Input: part model. Units: mm. Frame: model coordinates. Face numbers are marked on the shaded views. A direction names the side the tool comes from. Give positions to 0.01 mm unless a question says otherwise; leave off trailing zeros. Loops run counter-clockwise (first coordinate to the right, second up) from the corner with the lowest first, then second, coordinate; pieces in that order, holes last. Notation, with made-up numbers: M -6.5,-16.5 L 40.5,-16.5 A25 cw 40.5,22.5 Z; hole C 69,-7 d3. An arc over 180 degrees is marked long. Answer as a JSON object with one key per item and string values. Group by question number.
1) First-contact query: P1, Ø1, axis at x = 7.5, y = 3.5, coming from the -Z side; P2, Ø2.5, axis at x = -12.5, z = 0, coming from the -Y side. Flat tips, straight axial feed; report the tip coordinate or a pass-through.
2) Section query A-A on x = -12.5. Return loops of the section in (y, z).
3) Ray query, L1, parallel to X at y = 2, z = 0; L2, parallel to X at y = 2.65, z = 1; L3, parallel to X at y = 1.55, z = -3. Return the intervals inside material, ascending.
4) Draft query along X for the marked faces 4 and 5. Return one class per face: +X half, -X half, draft (parallel to the pull), parting line (faces both ways), or undercut.
5) Access query for the marked faces 1, 2 and 3. Directions: +Z, -Z, +X, -X, +Y, -Y. A direction counts if a zero-diameter tool reaches every point of the face in a straight line with its end or side. Return the directions, or none.
6) Section query C-C on y = 2. Return loops of the section in (x, z), plus the area to 3 significant figures.
7) Section query D-D on z = 4.75. Return loops of the section in (x, y), plus the area to 3 significant figures.
8) Section query B-B on z = 0. Return loops of the section in (x, y).
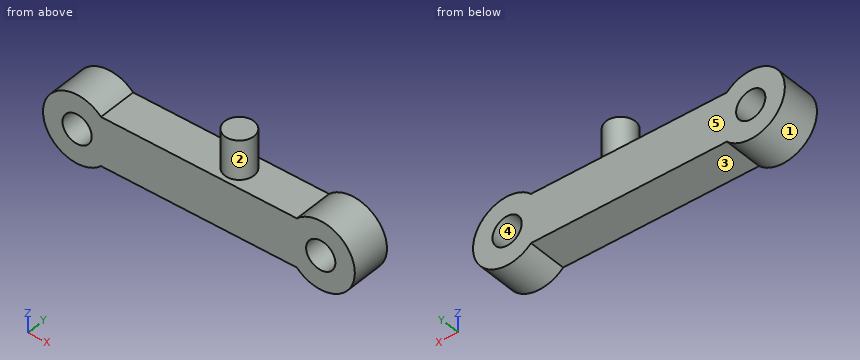
from build123d import *

# Parameters (mm, degrees)
SKETCH_1_R      = 1.5
EXTRUDE_1_DEPTH = 4
SKETCH_2_R      = 1.5
EXTRUDE_2_DEPTH = 4


with BuildPart() as part:
    # Эскиз1 → Бобышка-Вытянуть1 (new body)
    with BuildSketch(Plane(origin=(0, 0, 0), x_dir=(1, 0, 0), z_dir=(0, 1, 0))):
        with BuildLine():
            Line((-10.050510257, -2.5), (10.050510257, -2.5))
            ThreePointArc((10.050510257, -2.5), (16, 0), (10.050510257, 2.5))
            Line((10.050510257, 2.5), (-10.050510257, 2.5))
            ThreePointArc((-10.050510257, 2.5), (-16, 0), (-10.050510257, -2.5))
        make_face()
        with Locations(Location((-12.5, 0, 0), (0, 0, 270))):
            Circle(SKETCH_1_R, mode=Mode.SUBTRACT)
        with Locations(Location((12.5, 0, 0), (0, 0, 270))):
            Circle(SKETCH_1_R, mode=Mode.SUBTRACT)
    extrude(amount=EXTRUDE_1_DEPTH)

    # Эскиз2 → Бобышка-Вытянуть2 (add)
    with BuildSketch(Plane.XY.offset(2.5)):
        with Locations(Location((2.5, 2, 0), (0, 0, 180))):
            Circle(SKETCH_2_R)
    extrude(amount=EXTRUDE_2_DEPTH)


solid = part.part
Output:
{
 "1": {"P1": "stops at z = -2.5", "P2": "passes through"},
 "2": {"outline": "M 0,-3.5 L 4,-3.5 L 4,-1.5 L 0,-1.5 Z; M 0,1.5 L 4,1.5 L 4,3.5 L 0,3.5 Z"},
 "3": {"L1": "x = -16 to -14, -11 to 11, 14 to 16", "L2": "x = -15.85 to -13.62, -11.38 to 11.38, 13.62 to 15.85", "L3": "x = -14.3 to -10.7, 10.7 to 14.3"},
 "4": {"face 4": "undercut", "face 5": "draft"},
 "5": {"face 1": "+Y, -Y", "face 2": "+Z", "face 3": "-Z, +Y, -Y"},
 "6": {"outline": "M -10.05,-2.5 L 10.05,-2.5 A3.5 ccw long 10.05,2.5 L 4,2.5 L 4,6.5 L 1,6.5 L 1,2.5 L -10.05,2.5 A3.5 ccw long Z; hole C -12.5,0 d3; hole C 12.5,0 d3", "area": "168 mm^2"},
 "7": {"outline": "C 2.5,2 d3", "area": "7.07 mm^2"},
 "8": {"outline": "M -16,0 L -14,0 L -14,4 L -16,4 Z; M -11,0 L 11,0 L 11,4 L -11,4 Z; M 14,0 L 16,0 L 16,4 L 14,4 Z"}
}
